Autodesk Inventor part; units mm, degrees
ref_plane "YZ Plane" through (0, 0, 0) normal (1, 0, 0) x (0, 1, 0)
ref_plane "XZ Plane" through (0, 0, 0) normal (0, 1, 0) x (-1, 0, 0)
ref_plane "XY Plane" through (0, 0, 0) normal (0, 0, 1) x (1, 0, 0)
sketch "Sketch1" plane through (0, 0, 0) normal (0, 0, 1) x (1, 0, 0)
  line L0 (-125, -75) -> (125, -75)
  line L1 (125, -75) -> (125, 75)
  line L2 (125, 75) -> (-125, 75)
  line L3 (-125, 75) -> (-125, -75)
  line L4 (-125, -75) -> (125, 75) construction
  line L5 (125, -75) -> (-125, 75) construction
  point P0 (0, 0)
  dimension "d0" = 250
  dimension "d1" = 150
extrude "Extrusion1" add sketch "Sketch1" along normal blind 5
sketch "Sketch2" plane through (0, 0, 5) normal (0, 0, 1) x (1, 0, 0)
  line L0 (125, -75) -> (125, 75)
  line L1 (125, 75) -> (-125, 75)
  line L2 (-125, 75) -> (-125, -75)
  line L3 (-125, -75) -> (125, -75)
  line L4 (-120, 70) -> (120, 70)
  line L5 (120, 70) -> (120, -70)
  line L6 (120, -70) -> (-120, -70)
  line L7 (-120, -70) -> (-120, 70)
  point P0 (0, 0)
  dimension "d4" = 5
extrude "Extrusion2" add sketch "Sketch2" along normal blind 30
sketch "Sketch3" plane through (0, 0, 5) normal (0, 0, 1) x (1, 0, 0)
  line L0 (-120, 70) -> (-120, -70)
  line L1 (-120, -70) -> (120, -70)
  line L2 (120, -70) -> (120, 70)
  line L3 (120, 70) -> (-120, 70)
  circle A0 centre (0, 0) radius 18.5
  dimension "d8" = 37
extrude "Extrusion3" cut sketch "Sketch3" against normal through all contours A0
sketch "Sketch4" plane through (0, 0, 0) normal (0, 0, -1) x (-1, 0, 0)
  circle A0 centre (-65, 0) radius 18.5
  circle A1 centre (60, 0) radius 18.5
  line L0 (125, 75) -> (125, -75)
  line L1 (-125, -75) -> (-125, 75)
  line L2 (125, -75) -> (-125, -75)
  point P0 (0, 0)
  dimension "d15" = 37
  dimension "d16" = 37
  dimension "d17" = 125
  dimension "d18" = 65
  dimension "d19" = 60
  dimension "d20" = 75
extrude "Extrusion4" cut sketch "Sketch4" against normal through all
sketch "Sketch5" plane through (0, 0, 0) normal (0, 0, -1) x (-1, 0, 0)
  point P0 (0, 0)
properties part number "casing"
Design review of the part built by this model. Coordinates are the model's own, in mm. A direction names the side the tool comes from. Give positions to 0.01 mm unless a question says otherwise; leave off trailing zeros. Order: outer loops, then holes, each group sorted by start corner. A loop starts at its lowest first (then second) coordinate and runs counter-clockwise, first axis right, second up. Notation, with made-up numbers: (-35.75, -8.75) - (-12.75, -8.75) arc R22 ccw to (-12.75, 18.25) - close; hole circle Ø1 at (-40, 57.5). An arc over 180 degrees is marked (long way). Use CSV: the item, a comma, the result in double quotes. Start each with the question number.
Q1. For line 1 (X direction, y = -9, z = 16); line 2 (Y direction, x = 94, z = 15); line 3 (Y direction, x = -60, z = 2.15), list the stretches that pass through material, from the lowest coordinate up.
Q2. Draft analysis for pull direction Y (two halves, no side actions). For faces 3 (the face through (-2, -75, 17)), 4 (the face through (2, 75, 17)), 5 (the face through (25, 1, 5)), state which applies: pulls with the +Y half, pulls with the -Y half, needs draft (parallel to the pull), parting line crosses it, or undercut.
Q3. For P1, Ø12, axis at x = 90, y = -49, coming from the +Z side, flat-tipped, find the tip position at first contact; note if it passes through.
Q4. Take a section at D-D (x = -86.5). State the section outline as (y, z) points, and give its area (3 significant figures).
Q5. Take a section at A-A (z = 30.5). State the section outline as (x, y) points.
Q6. Take a section at B-B (x = 0). State the section outline as (y, z) points, and give its area (3 significant figures).
Q7. Take a section at C-C (y = 0). State the section outline as (x, z) points.
Q8. Machinability: for faces 1 (the face through (120, 1, 20)), 2 (the face through (-4.01, -18.06, 2.54)), which of the approach directions +Z, -Z, +X, -X, +Y, -Y give a long, thin tool a straight path to every point of the face, cutting with its end or side? Answer none if there is none.
Calculated:
1,line 1,"x = -125 to -120, 120 to 125"
1,line 2,"y = -75 to -70, 70 to 75"
1,line 3,"y = -75 to -18.5, 18.5 to 75"
2,face 3,"pulls with the -Y half"
2,face 4,"pulls with the +Y half"
2,face 5,"undercut"
3,P1,"stops at z = 5"
4,outline,"(-75, 0) - (75, 0) - (75, 35) - (70, 35) - (70, 5) - (-70, 5) - (-70, 35) - (-75, 35) - close"
4,area,"1,050 mm²"
5,outline,"(-125, -75) - (125, -75) - (125, 75) - (-125, 75) - close; hole (-120, -70) - (120, -70) - (120, 70) - (-120, 70) - close"
6,outline,"(-75, 0) - (-18.5, 0) - (-18.5, 5) - (-70, 5) - (-70, 35) - (-75, 35) - close; (18.5, 0) - (75, 0) - (75, 35) - (70, 35) - (70, 5) - (18.5, 5) - close"
6,area,"865 mm²"
7,outline,"(-125, 0) - (-78.5, 0) - (-78.5, 5) - (-120, 5) - (-120, 35) - (-125, 35) - close; (-41.5, 0) - (-18.5, 0) - (-18.5, 5) - (-41.5, 5) - close; (18.5, 0) - (46.5, 0) - (46.5, 5) - (18.5, 5) - close; (83.5, 0) - (125, 0) - (125, 35) - (120, 35) - (120, 5) - (83.5, 5) - close"
8,face 1,"+Z"
8,face 2,"+Z, -Z"
